Job drawing, mm, ordinate dimensions from the low corner. One solid piece. A direction names the side the tool comes from. Give positions to 0.01 mm unless a question says otherwise; leave off trailing zeros. Loops run counter-clockwise (first coordinate to the right, second up) from the corner with the lowest first, then second, coordinate; pieces in that order, holes last. Notation, with made-up numbers: M -13.75,12.25 L 30.25,12.25 A18 ccw 30.25,31.25 Z; hole C 19.5,-16.5 d2. An arc over 180 degrees is marked long. Put each result on its own line as item: value.
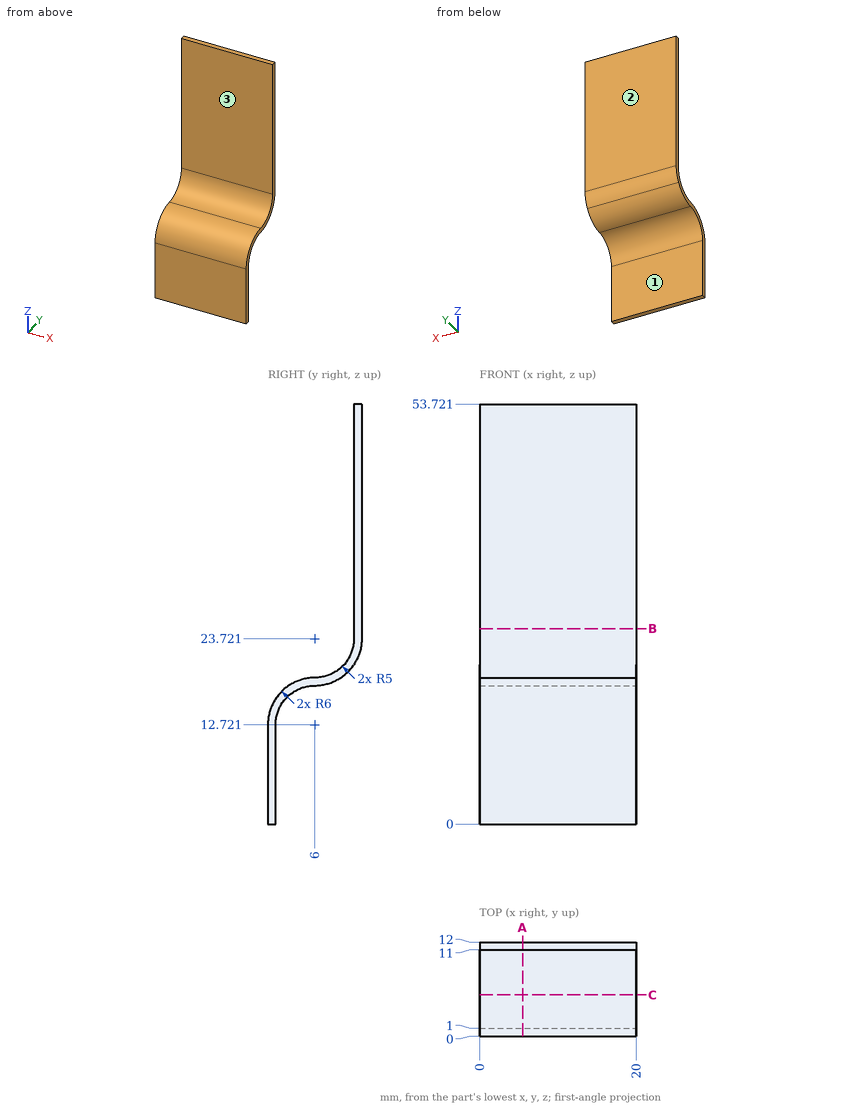
Q1. Slice it at C-C (y = 5.25). List the corners of the cut face in (x, z) (1 decimal).
Here are the results:
outline: M 0,17.7 L 20,17.7 L 20,18.7 L 0,18.7 Z
Q2. Drop flat-ended pins along their axis: pin 1 Ø6 at (x, z) = (8.5, 11) entering from +Y; pin 2 Ø6 at (x, z) = (6.5, 41.5) entering from -Y; pin 3 Ø3 at (x, z) = (7.5, 6) entering from +Y. Give the stop position or say it passes through.
Here are the results:
pin 1: y = 1.17
pin 2: y = 11
pin 3: y = 1
Q3. Slice it at A-A (x = 5.5). List the corners of the cut face in (y, z) (1 decimal).
Here are the results:
outline: M 0,0 L 1,0 L 1,12.7 A5 cw 6,17.7 A6 ccw 12,23.7 L 12,53.7 L 11,53.7 L 11,23.7 A5 cw 6,18.7 A6 ccw 0,12.7 Z
Q4. Probe line 1 (Y direction, x = 7.25, z = 42.5); line 2 (Z direction, x = 11.5, y = 6); line 3 (Y direction, x = 12, z = 6). List the from-to ranges inside material, lowest first. Write a range as from..to.
Here are the results:
line 1: 11..12
line 2: 17.72..18.72
line 3: 0..1
Q5. Slice it at B-B (z = 25). List the corners of the cut face in (x, y).
Here are the results:
outline: M 0,11 L 20,11 L 20,12 L 0,12 Z
Q6. Tool access for the marked faces 1, 2 and 3: list every direction of +Z, -Z, +X, -X, +Y, -Y with a clear straight run to the whole face (end or side of a thin tool).
Here are the results:
face 1: -Z, +X, -X, +Y
face 2: +Z, -Z, +X, -X, +Y
face 3: +Z, +X, -X, -Y
